Part model, mm, in its own coordinate system. Face numbers are marked on the shaded views. A direction names the side the tool comes from. Round coordinates to 2 decimals unless told otherwise and drop trailing zeros. Write each loop counter-clockwise with the first axis right and the second up, starting at its lowest first coordinate (ties: lowest second). Pieces come first, ordered by that corner, then holes.
1) Which spindle directions (+Z, -Z, +X, -X, +Y, -Y) get a long thin tool onto all of the face, cutting with end or side? Do the marked faces 1 and 2. Say none if no direction does.
2) Saw through at A-A on z = 0. Write the cut outline in (x, y), and give its area (3 significant figures).
3) Flat gauge pins, fed straight in: pin 1 (6 mm diameter, centred on x = 18.5, z = -30.5, fed in from -Y); pin 2 (2 mm diameter, centred on x = 13, z = -30.5, fed in from +Y). Where does each tip first touch, or does it go through?
4) Saw through at C-C on y = 14. Write the cut outline in (x, z).
5) Drill centre lines: L1, parallel to Y at x = 4.5, z = 28.5; L2, parallel to X at y = 16.5, z = -4; L3, parallel to Y at x = 21, z = -1. Where is each one in solid material? Low to high.
6) Saw through at B-B on x = 0. Write the cut outline in (y, z), and give its area (3 significant figures).
7) Saw through at D-D on z = -27.5. Write the cut outline in (x, y), and give its area (3 significant figures).
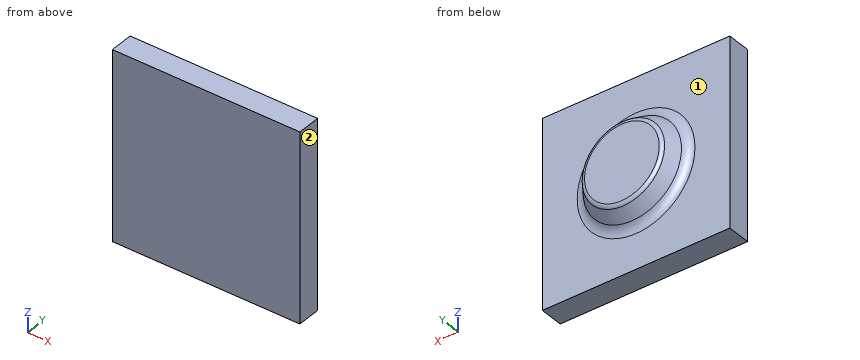
```python
from build123d import *

# Parameters (mm, degrees)
SKETCH_1_W      = 80
SKETCH_1_H      = 80
EXTRUDE_1_DEPTH = 10
FILLET_1_R      = 5
FILLET_2_R      = 2


with BuildPart() as part:
    # 草图1 → 凸台-拉伸1 (new body)
    with BuildSketch(Plane(origin=(0, 0, 0), x_dir=(1, 0, 0), z_dir=(0, 1, 0))):
        Rectangle(SKETCH_1_W, SKETCH_1_H)
    extrude(amount=EXTRUDE_1_DEPTH)

    # 草图2 → 旋转1 (revolve)
    with BuildSketch(Plane.XY):
        Polygon((0, 18), (0, 10), (22.5, 10), (17, 18), align=None)
    revolve(axis=Axis((0, 0, 0), (0, 1, 0)))

    # 圆角1
    fillet_1_edges = [part.edges().sort_by_distance(p)[0] for p in [
        (-22.5, 10, 0),
    ]]
    fillet(fillet_1_edges, radius=FILLET_1_R)

    # 圆角2
    fillet_2_edges = [part.edges().sort_by_distance(p)[0] for p in [
        (-17, 18, 0),
    ]]
    fillet(fillet_2_edges, radius=FILLET_2_R)


solid = part.part
```
Completed:
1. face 1: +Y
1. face 2: +Z, -Z, +X, +Y, -Y
2. outline: (-40, 0) - (40, 0) - (40, 10) - (25.13, 10) arc R5 cw to (21.01, 12.17) - (17.6, 17.13) arc R2 ccw to (15.95, 18) - (-15.95, 18) arc R2 ccw to (-17.6, 17.13) - (-21.01, 12.17) arc R5 cw to (-25.13, 10) - (-40, 10) - close
2. area: 1,120 mm2
3. pin 1: stops at y = 0
3. pin 2: stops at y = 10
4. outline: circle Ø39.5 at (0, 0)
5. L1: y = 0 to 10
5. L2: x = -17.58 to 17.58
5. L3: y = 0 to 12.15
6. outline: (0, -40) - (10, -40) - (10, -25.13) arc R5 cw to (12.17, -21.01) - (17.13, -17.6) arc R2 ccw to (18, -15.95) - (18, 15.95) arc R2 ccw to (17.13, 17.6) - (12.17, 21.01) arc R5 cw to (10, 25.13) - (10, 40) - (0, 40) - close
6. area: 1,120 mm2
7. outline: (-40, 0) - (40, 0) - (40, 10) - (-40, 10) - close
7. area: 800 mm2
